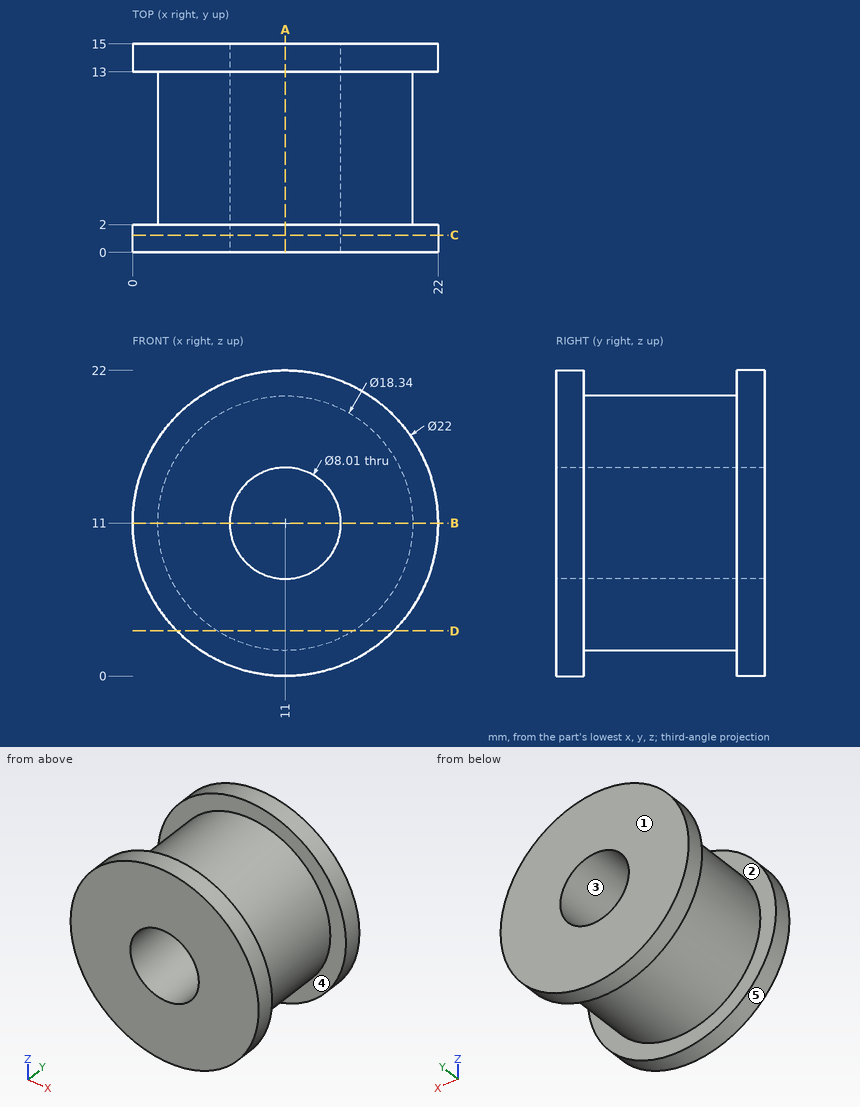
Could you check a few things on this drawing? It's one solid part, dimensions in mm from its lowest x, y, z. A direction names the side the tool comes from. Give positions to 0.01 mm unless a question says otherwise; leave off trailing zeros. Loops run counter-clockwise (first coordinate to the right, second up) from the corner with the lowest first, then second, coordinate; pieces in that order, holes last. Notation, with made-up numbers: M 50,-38 L 99,-38 A30 ccw 99,-14 Z; hole C 45.5,27 d10. An arc over 180 degrees is marked long. Return JSON: item names as keys, results as strings.
Item 1: On a 3-axis mill with a long thin cutter (end or side, diameter ignored), from which of +Z, -Z, +X, -X, +Y, -Y can I reach the whole of each face in a straight line? I mean the marked faces 1 and 2. Say none if no direction works.
A:
{"face 1": "+Z, -Z, +X, -X, +Y", "face 2": "none"}
Item 2: Imagine slicing it at A-A on x = 11. List the corners of the cut face in (y, z) for me (3 decimals), then the cut area to 3 significant figures.
A:
{"outline": "M 0,0 L 2,0 L 2,1.83 L 13,1.83 L 13,0 L 15,0 L 15,6.995 L 0,6.995 Z; M 0,15.005 L 15,15.005 L 15,22 L 13,22 L 13,20.17 L 2,20.17 L 2,22 L 0,22 Z", "area": "170 mm^2"}
Item 3: Thinking about a two-plate mould opening in X: for the marked faces 3, 4 and 5, which applies, released by +X, released by -X, zero draft, split by the parting line, or undercut?
A:
{"face 3": "undercut", "face 4": "zero draft", "face 5": "split by the parting line"}
Item 4: Imagine slicing it at C-C on y = 1.25. List the corners of the cut face in (x, z) for me (3 decimals).
A:
{"outline": "C 11,11 d22; hole C 11,11 d8.01"}
Item 5: Imagine slicing it at B-B on z = 11. List the corners of the cut face in (x, y) for me (3 decimals), then the cut area to 3 significant figures.
A:
{"outline": "M 0,0 L 6.995,0 L 6.995,15 L 0,15 L 0,13 L 1.83,13 L 1.83,2 L 0,2 Z; M 15.005,0 L 22,0 L 22,2 L 20.17,2 L 20.17,13 L 22,13 L 22,15 L 15.005,15 Z", "area": "170 mm^2"}
Item 6: Please list where these lines run through material, in increasing order: line 1 (Z direction, x = 11, y = 11.75) (3 decimals); line 2 (Y direction, x = 18.5, z = 18); line 3 (X direction, y = 3.75, z = 13).
A:
{"line 1": "z = 1.83 to 6.995, 15.005 to 20.17", "line 2": "y = 0 to 2, 13 to 15", "line 3": "x = 2.05 to 7.53, 14.47 to 19.95"}
Item 7: I'm going to push flat-ended pins straight in: pin 1 Ø6 at (y, z) = (11.5, 16) entering from -X; pin 2 Ø5 at (y, z) = (8.5, 6.5) entering from +X; pin 3 Ø3 at (x, y) = (9, 5.5) entering from +Z. Where does each tip first touch, or does it pass through?
A:
{"pin 1": "stops at x = 0.27", "pin 2": "stops at x = 19.95", "pin 3": "stops at z = 20.16"}
Item 8: Imagine slicing it at D-D on z = 3.25. List the corners of the cut face in (x, y) for me, then the cut area to 3 significant figures.
A:
{"outline": "M 3.19,0 L 18.81,0 L 18.81,2 L 15.9,2 L 15.9,13 L 18.81,13 L 18.81,15 L 3.19,15 L 3.19,13 L 6.1,13 L 6.1,2 L 3.19,2 Z", "area": "170 mm^2"}
